Study the drawing (mm; zero at the part's minimum x, y, z) and answer. Round coordinates to 2 decimals unless told otherwise and drop trailing zeros. Loops run counter-clockwise (first coordinate to the right, second up) from the corner with the lowest first, then second, coordinate; pieces in that order, holes last. Notation, with made-up numbers: (-1.5, 58) -> (17.5, 58) arc R29 cw to (17.5, 80) -> close; hole circle Ø1 at (26, 44.5). An arc over 180 degrees is marked (long way). Use one line per item in the form item = value.
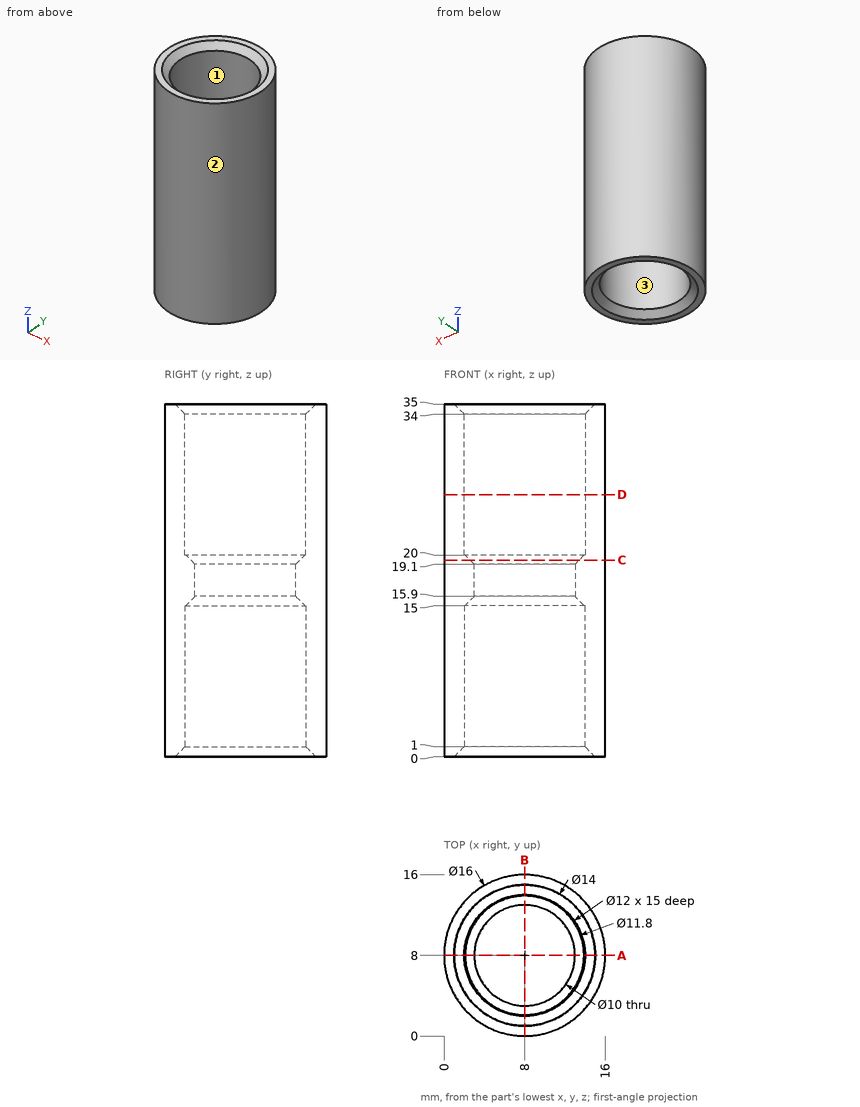
(1) Given P1, Ø1.5, axis at x = 2, y = 8, coming from the +Z side; P2, Ø9.5, axis at x = 8, y = 8, coming from the +Z side; P3, Ø3, axis at y = 3, z = 8, coming from the -X side; P4, Ø6, axis at x = 10, y = 7.5, coming from the -Z side, each flat-ended and moving along its own axis, determine where each tip first touches the part or whether it passes through.
Completed:
P1 = 34.75
P2 = through
P3 = 0.81
P4 = 15.84
(2) Consider L1, parallel to Y at x = 8, z = 17.9; L2, parallel to Y at x = 8, z = 30; L3, parallel to X at y = 10.75, z = 9.5. Determine where each line is inside the solid, lowest interval first.
Completed:
L1 = 0 to 3, 13 to 16
L2 = 0 to 2, 14 to 16
L3 = 0.49 to 2.67, 13.33 to 15.51
(3) For a pull along X with two mould halves and no side action, classify the marked faces 1, 2 and 3 as +X half, -X half, draft (parallel to the pull), parting line (faces both ways), or undercut.
Completed:
face_1 = undercut
face_2 = parting line
face_3 = undercut
(4) Find section A-A, the plane y = 8. Write down the section's boundary in (x, z).
Completed:
outline = (0, 0) -> (1, 0) -> (2, 1) -> (2, 15) -> (2.1, 15) -> (3, 15.9) -> (3, 19.1) -> (2.1, 20) -> (2, 20) -> (2, 34) -> (1, 35) -> (0, 35) -> close; (13, 15.9) -> (13.9, 15) -> (14, 15) -> (14, 1) -> (15, 0) -> (16, 0) -> (16, 35) -> (15, 35) -> (14, 34) -> (14, 20) -> (13.9, 20) -> (13, 19.1) -> close
(5) Find section C-C, the plane z = 19.5. Write down the section's boundary in (x, y), then the cut area to 3 significant figures.
Completed:
outline = circle Ø16 at (8, 8); hole circle Ø10.8 at (8, 8)
area = 109 mm2
(6) Find section D-D, the plane z = 26. Write down the section's boundary in (x, y).
Completed:
outline = circle Ø16 at (8, 8); hole circle Ø12 at (8, 8)
